Here's how the part is built. I have some questions about the finished solid (model axes, mm). Coordinates: 2 decimals unless noted, no trailing zeros. Write each loop counter-clockwise with the first axis right and the second up, starting at its lowest first coordinate (ties: lowest second). Pieces come first, ordered by that corner, then holes. Notation, with made-up numbers: (75.25, -25.75) - (80.25, -25.75) arc R20 cw to (80.25, -11.75) - close; hole circle Ø6 at (44, 89.25). An arc over 180 degrees is marked (long way). Answer in a Markdown table with one row per item. Add a question column.
Item 1: Imagine slicing it at A-A (z = 325.4). Please give me the cut outline in (x, y), plus the area to 3 significant figures.
Item 2: Imagine slicing it at B-B (y = -155.5). Please give me the cut outline in (x, z), plus the area to 3 significant figures.
Item 3: Imagine slicing it at C-C (x = 426). Please give me the cut outline in (y, z).
Item 4: If I drill on probe 1 along Y at (x, z) = (431.25, 325.7); probe 2 along X at (y, z) = (-150, 325.55), over which ranges is the centre line in solid material (lowest first)? Write a range as from..to.
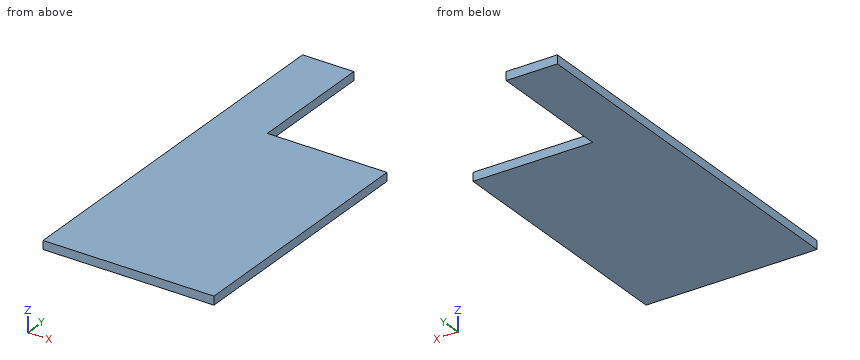
from build123d import *

# Parameters (mm, degrees)
BOX007_W           = 10
BOX007_H           = 15
BOX007_DEPTH       = 14
BOX006_W           = 1
BOX006_H           = 45
BOX006_DEPTH       = 20
CUT006_PITCH_ANGLE = 90


with BuildPart() as cubo005:
    # Box007 → Box007 (new body)
    with BuildSketch(Plane(origin=(-4, -227, 60), x_dir=(1, 0, 0), z_dir=(0, 0, 1))):
        with Locations((5, 7.5)):
            Rectangle(BOX007_W, BOX007_H)
    extrude(amount=BOX007_DEPTH)


with BuildPart() as cut006:
    # Box006 → Box006 (new body)
    with BuildSketch(Plane(origin=(0, -257, 54), x_dir=(1, 0, 0), z_dir=(0, 0, 1))):
        with Locations((0.5, 22.5)):
            Rectangle(BOX006_W, BOX006_H)
    extrude(amount=BOX006_DEPTH)

    # Cut006: cut Cubo005
    add(cubo005.part, mode=Mode.SUBTRACT)


with BuildPart() as cut006_1:
    # Cut006 pitch: moved
    add(cut006.part.rotate(Axis((0, 0, 0), (0, 1, 0)), CUT006_PITCH_ANGLE))


with BuildPart() as cut006_2:
    # Cut006 placement: moved
    add(cut006_1.part.moved(Location((359, 67, 326))))


solid = cut006_2.part
Here are the results:
| question | item | result |
|---|---|---|
| 1 | outline | (413, -190) - (433, -190) - (433, -160) - (419, -160) - (419, -145) - (413, -145) - close |
| 1 | area | 690 mm2 |
| 2 | outline | (413, 325) - (419, 325) - (419, 326) - (413, 326) - close |
| 2 | area | 6.00 mm2 |
| 3 | outline | (-190, 325) - (-160, 325) - (-160, 326) - (-190, 326) - close |
| 4 | probe 1 | y = -190..-160 |
| 4 | probe 2 | x = 413..419 |
